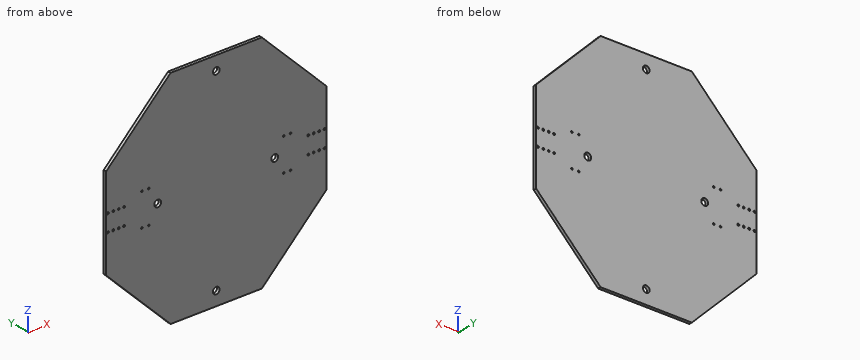
Autodesk Inventor part; units mm, degrees
ref_plane "YZ Plane" through (0, 0, 0) normal (1, 0, 0) x (0, 1, 0)
ref_plane "XZ Plane" through (0, 0, 0) normal (0, 1, 0) x (-1, 0, 0)
ref_plane "XY Plane" through (0, 0, 0) normal (0, 0, 1) x (1, 0, 0)
sketch "Sketch1" plane through (0, 0, 0) normal (0, 1, 0) x (-1, 0, 0)
  line L0 (-203.2, 84.1682) -> (-84.1682, 203.2)
  line L1 (-84.1682, 203.2) -> (84.1682, 203.2)
  line L2 (84.1682, 203.2) -> (203.2, 84.1682)
  line L3 (203.2, 84.1682) -> (203.2, -84.1682)
  line L4 (203.2, -84.1682) -> (84.1682, -203.2)
  line L5 (84.1682, -203.2) -> (-84.1682, -203.2)
  line L6 (-84.1682, -203.2) -> (-203.2, -84.1682)
  line L7 (-203.2, -84.1682) -> (-203.2, 84.1682)
  point P0 (0, 0)
  point P1 (0, 0)
  dimension "BaseWidth" = 406.4
  dimension "BaseSideLength" = 168.3364
extrude "Extrusion1" add sketch "Sketch1" along normal blind 5.5563
sketch "Sketch2" plane through (0, 5.5563, 0) normal (0, 1, 0) x (1, 0, 0)
  line L0 (84.1682, -203.2) -> (-84.1682, -203.2)
  line L1 (203.2, 84.1682) -> (203.2, -84.1682)
  line L2 (-203.2, -84.1682) -> (-203.2, 84.1682)
  line L3 (84.1682, -203.2) -> (-84.1682, -203.2)
  line L4 (203.2, 84.1682) -> (203.2, -84.1682)
  line L5 (-84.1682, 203.2) -> (84.1682, 203.2)
  line L6 (-203.2, -84.1682) -> (-203.2, 84.1682)
  line L7 (-203.2, 0) -> (203.2, 0)
  line L8 (0, 203.2) -> (0, -203.2)
  circle A0 centre (-170.025, 15.5) radius 1.75
  circle A1 centre (-180.025, 15.5) radius 1.75
  circle A2 centre (-190.025, 15.5) radius 1.75
  circle A3 centre (-200.025, 15.5) radius 1.75
  circle A4 centre (-170.025, -15.5) radius 1.75
  circle A5 centre (-180.025, -15.5) radius 1.75
  circle A6 centre (-190.025, -15.5) radius 1.75
  circle A7 centre (-200.025, -15.5) radius 1.75
  circle A8 centre (170.025, 15.5) radius 1.75
  circle A9 centre (180.025, 15.5) radius 1.75
  circle A10 centre (190.025, 15.5) radius 1.75
  circle A11 centre (200.025, 15.5) radius 1.75
  circle A12 centre (170.025, -15.5) radius 1.75
  circle A13 centre (180.025, -15.5) radius 1.75
  circle A14 centre (190.025, -15.5) radius 1.75
  circle A15 centre (200.025, -15.5) radius 1.75
  circle A16 centre (0, -177.8) radius 6.1516
  circle A17 centre (0, 177.8) radius 6.1516
  circle A18 centre (-107.95, 0) radius 6.35
  circle A19 centre (107.95, 0) radius 6.35
  dimension "d39" = 3.5
  dimension "d42" = 10
  dimension "d45" = 31
  dimension "d48" = 3.5
  dimension "d51" = 10
  dimension "d54" = 31
  dimension "d57" = 15.5
  dimension "d58" = 3.175
  dimension "d59" = 3.175
  dimension "d60" = 15.5
  dimension "d71" = 12.3031
  dimension "d72" = 12.3031
  dimension "d73" = 25.4
  dimension "d74" = 25.4
  dimension "d75" = 12.7
  dimension "d76" = 95.25
  dimension "d77" = 95.25
extrude "Extrusion2" cut sketch "Sketch2" against normal through all
sketch "Sketch3" plane through (0, 5.5563, 0) normal (0, 1, 0) x (1, 0, 0)
  line L0 (84.1682, -203.2) -> (-84.1682, -203.2)
  line L1 (203.2, -84.1682) -> (84.1682, -203.2)
  line L2 (203.2, 84.1682) -> (203.2, -84.1682)
  line L3 (84.1682, 203.2) -> (203.2, 84.1682)
  line L4 (-84.1682, 203.2) -> (84.1682, 203.2)
  line L5 (-203.2, 84.1682) -> (-84.1682, 203.2)
  line L6 (-203.2, -84.1682) -> (-203.2, 84.1682)
  line L7 (-84.1682, -203.2) -> (-203.2, -84.1682)
  line L8 (-203.2, 0) -> (203.2, 0)
  line L9 (0, 203.2) -> (0, -203.2)
  point P0 (0, 0)
sketch "Sketch5" plane through (0, 5.5563, 0) normal (0, 1, 0) x (1, 0, 0)
  circle A0 centre (-107.95, 0) radius 6.35
  line L0 (84.1682, -203.2) -> (-84.1682, -203.2)
  line L1 (203.2, 84.1682) -> (203.2, -84.1682)
  line L2 (-203.2, -84.1682) -> (-203.2, 84.1682)
  circle A1 centre (-137.16, 29.8379) radius 1.5
  circle A2 centre (-124.46, 29.8379) radius 1.5
  circle A3 centre (-137.16, -29.8379) radius 1.5
  circle A4 centre (-124.46, -29.8379) radius 1.5
  point P0 (0, 0)
  dimension "d78" = 66.04
  dimension "d80" = 3
  dimension "d81" = 29.8379
  dimension "d84" = 12.7
  dimension "d87" = 59.6758
extrude "Extrusion4" cut sketch "Sketch5" against normal through all contours A1 | A2 | A3 | A4
mirror "Mirror1" about plane through (0, 0, 0) normal (1, 0, 0) of "Extrusion4"
equation "\"d71\" = CasterDrillDiameter"
equation "\"d72\" = CasterDrillDiameter"
equation "\"d77\" = d76"
equation "\"d80\" = HoleDiameter"
equation "\"d81\" = 0.5 * ShroudHoldLongSeperation"
equation "\"d84\" = ShroudHoldShortSeperation"
equation "\"d87\" = ShroudHoldLongSeperation"
equation "\"BaseSupportThickness\" = 12.7"
equation "\"CasterDrillDiameter\" = 12.30312"
properties part number "Robot-Lower-Base" material "Wood (Birch)"
Input: part model. Units: mm. Frame: model coordinates. Coordinates: 2 decimals unless noted, no trailing zeros. Loops run counter-clockwise (first coordinate to the right, second up) from the corner with the lowest first, then second, coordinate; pieces in that order, holes last.
Q1. Section D-D, the plane x = 107.95. Return the cut outline in (y, z).
Results are:
outline: (0, -179.42) - (5.56, -179.42) - (5.56, -6.35) - (0, -6.35) - close; (0, 6.35) - (5.56, 6.35) - (5.56, 179.42) - (0, 179.42) - close
Q2. Section B-B, the plane x = 0. Return the cut outline in (y, z), and give its area (3 significant figures).
Results are:
outline: (0, -203.2) - (5.56, -203.2) - (5.56, -183.95) - (0, -183.95) - close; (0, -171.65) - (5.56, -171.65) - (5.56, 171.65) - (0, 171.65) - close; (0, 183.95) - (5.56, 183.95) - (5.56, 203.2) - (0, 203.2) - close
area: 2,120 mm2
Q3. Line query: line 1 along Z through (x, y) = (-169, 2.25); line 2 along X through (y, z) = (1.35, 0); line 3 along Z through (x, y) = (107.95, 1.5). Output: solid intervals per line, ascending.
Results are:
line 1: z = -118.37 to -16.92, -14.08 to 14.08, 16.92 to 118.37
line 2: x = -203.2 to -114.3, -101.6 to 101.6, 114.3 to 203.2
line 3: z = -179.42 to -6.35, 6.35 to 179.42
Q4. Contact query for flat-ended pins moving along their axis: pin 1 (1.8 mm diameter, centred on x = 124.46, z = -29.84, fed in from +Y); pin 2 (2 mm diameter, centred on x = 94.5, y = 1, fed in from +Z); pin 3 (1.5 mm diameter, centred on y = 2.5, z = -152.5, fed in from -X). Output: stop coordinate, or through.
Results are:
pin 1: passes through
pin 2: stops at z = 193.87
pin 3: stops at x = -135.62
Q5. Section C-C, the plane z = 177.8. Return the cut outline in (x, y), and give its area (3 significant figures).
Results are:
outline: (-109.57, 0) - (-6.15, 0) - (-6.15, 5.56) - (-109.57, 5.56) - close; (6.15, 0) - (109.57, 0) - (109.57, 5.56) - (6.15, 5.56) - close
area: 1,150 mm2
Q6. Section A-A, the plane z = 0. Return the cut outline in (x, y).
Results are:
outline: (-203.2, 0) - (-114.3, 0) - (-114.3, 5.56) - (-203.2, 5.56) - close; (-101.6, 0) - (101.6, 0) - (101.6, 5.56) - (-101.6, 5.56) - close; (114.3, 0) - (203.2, 0) - (203.2, 5.56) - (114.3, 5.56) - close
